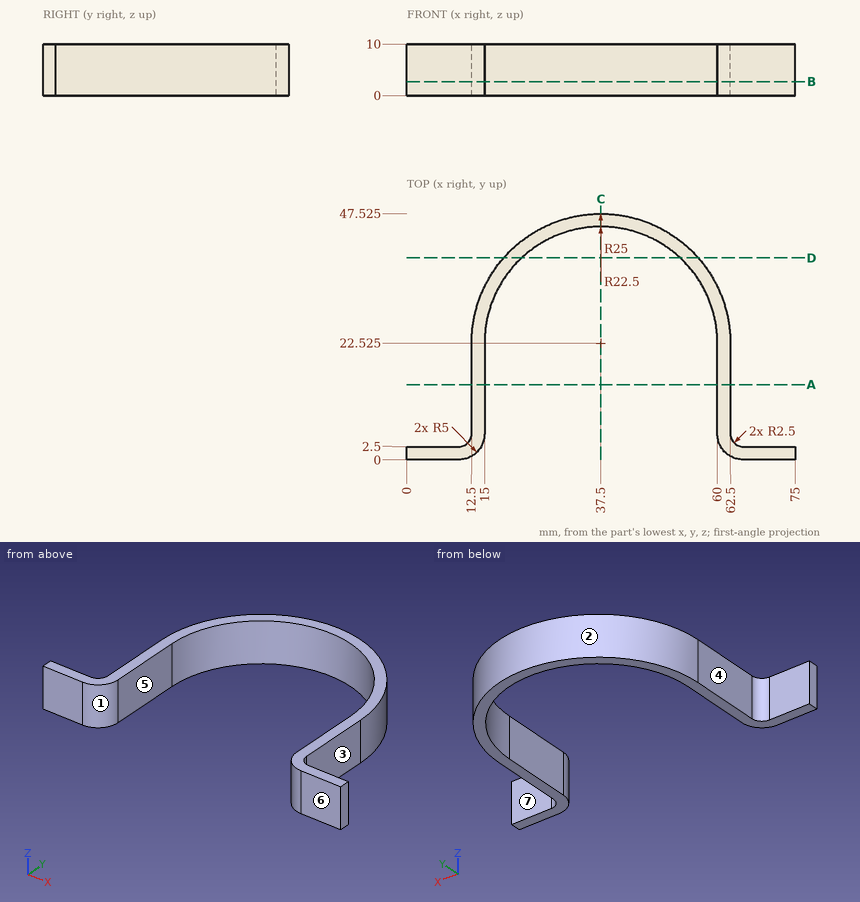
Could you check a few things on this drawing? It's one solid part, dimensions in mm from its lowest x, y, z. A direction names the side the tool comes from. Coordinates: 2 decimals unless noted, no trailing zeros. Order: outer loops, then holes, each group sorted by start corner. A loop starts at its lowest first (then second) coordinate and runs counter-clockwise, first axis right, second up. Notation, with made-up numbers: (45.25, 48.5) - (52.25, 48.5) arc R19 ccw to (52.25, 59.5) - close; hole circle Ø4 at (-25.75, 55). An arc over 180 degrees is marked (long way). Answer as a JSON object with one key per item and string values. Group by question number.
Q1. On a 3-axis mill with a long thin cutter (end or side, diameter ignored), from which of +Z, -Z, +X, -X, +Y, -Y can I reach the whole of each face in a straight line? I mean the marked faces 4, 5, 6 and 7. Say none if no direction works.
Q2. Imagine slicing it at B-B (z = 2.75). Please give me the cut outline in (x, y) (1 decimal).
Q3. Imagine slicing it at A-A (y = 14.5). Please give me the cut outline in (x, z).
Q4. Imagine slicing it at D-D (y = 39). Please give me the cut outline in (x, z).
Q5. Will these pins go through, and if not, where does the flat tip stop? P1, Ø2, axis at x = 67, z = 8.5, coming from the -Y side; P2, Ø5, axis at x = 70, z = 2.5, coming from the +Y side; P3, Ø3, axis at y = 15, z = 4.5, coming from the -X side; P4, Ø5, axis at y = 13, z = 4, coming from the +X side.
Q6. We'd pull the mould along X, two halves only. Please class the marked faces 1, 2 and 3: +X half, -X half, draft (parallel to the pull), parting line (faces both ways), or undercut.
Q7. I need wall thicknesses on line 1 (X direction, y = 19, z = 8); line 2 (Y direction, x = 7.5, z = 8.25); line 3 (X direction, y = 29.5, z = 8.75). Which ranges of each line are inside material? Lowest first, please. Write a range as from..to.
Q8. Imagine slicing it at C-C (x = 37.5). Please give me the cut outline in (y, z) (1 decimal), and give its area (3 significant figures).
Determined:
{
 "1": {"face 4": "+Z, -Z, -X, +Y", "face 5": "+Z, -Z, -Y", "face 6": "+Z, -Z, +X, -X, -Y", "face 7": "+Z, -Z, +X, +Y"},
 "2": {"outline": "(0, 0) - (10, 0) arc R5 ccw to (15, 5) - (15, 22.5) arc R22.5 cw to (60, 22.5) - (60, 5) arc R5 ccw to (65, 0) - (75, 0) - (75, 2.5) - (65, 2.5) arc R2.5 cw to (62.5, 5) - (62.5, 22.5) arc R25 ccw to (12.5, 22.5) - (12.5, 5) arc R2.5 cw to (10, 2.5) - (0, 2.5) - close"},
 "3": {"outline": "(12.5, 0) - (15, 0) - (15, 10) - (12.5, 10) - close; (60, 0) - (62.5, 0) - (62.5, 10) - (60, 10) - close"},
 "4": {"outline": "(18.7, 0) - (22.18, 0) - (22.18, 10) - (18.7, 10) - close; (52.82, 0) - (56.3, 0) - (56.3, 10) - (52.82, 10) - close"},
 "5": {"P1": "stops at y = 0", "P2": "stops at y = 2.5", "P3": "stops at x = 12.5", "P4": "stops at x = 62.5"},
 "6": {"face 1": "undercut", "face 2": "parting line", "face 3": "+X half"},
 "7": {"line 1": "x = 12.5..15, 60..62.5", "line 2": "y = 0..2.5", "line 3": "x = 13.49..16.11, 58.89..61.51"},
 "8": {"outline": "(45, 0) - (47.5, 0) - (47.5, 10) - (45, 10) - close", "area": "25.0 mm2"}
}
